Could you check a few things on this model? Use its own coordinates, in mm. Face numbers are marked on the shaded views. A direction names the side the tool comes from. Give positions to 0.01 mm unless a question says otherwise; leave off trailing zeros. Loops run counter-clockwise (first coordinate to the right, second up) from the corner with the lowest first, then second, coordinate; pieces in that order, holes last. Notation, with made-up numbers: M 55,27 L 109,27 A21 cw 109,35 Z; hole C 50.25,-16.75 d1. An arc over 180 degrees is marked long. Return JSON: item names as keys, results as strings. Group by question number.
1. For the marked faces 4 and 5, which set-ups out of +Z, -Z, +X, -X, +Y, -Y let a thin tool reach every point of the face, with its end or its side?
2. Please list where these lines run through material, in increasing order: line 1 (Z direction, x = 5.75, y = -4.75); line 2 (Z direction, x = -3, y = -7); line 3 (Z direction, x = 2.75, y = 11.5).
3. If we mould it in two halves opening along Z, with no side actions, what happens to the marked faces 1, 2 and 3? For each: +Z half, -Z half, draft (parallel to the pull), parting line (faces both ways), or undercut.
4. If we section it at A-A (z = 0.5): Write out the boundary of the cut face in (x, y), plus the area to 3 significant figures.
5. For pin 1 (1.4 mm diameter, centred on x = -11.5, y = 6, fed in from -Z); pin 2 (1.6 mm diameter, centred on x = -11.5, y = -6.5, fed in from -Z); pin 3 (0.8 mm diameter, centred on x = -7.5, z = -2, fed in from -Y); pin 4 (3 mm diameter, centred on x = -11, y = 6, fed in from +Z), each with a flat end and sliding along its axis, tell me the tip position at first contact or that it passes through.
```python
from build123d import *

# Parameters (mm, degrees)
EXTRUDE_1_DEPTH     = 9.5
SKETCH_6_R          = 7
EXTRUDE_2_DEPTH     = 13.5
SWEEP_1_PITCH       = 4
SWEEP_1_HEIGHT      = 10
SWEEP_1_RADIUS      = 7
REVOLVE_2_ANGLE     = 45
CHAMFER_1_SIZE      = 1
CUT_EXTRUDE_2_DEPTH = 0.4
SKETCH_13_R         = 2.5
CUT_EXTRUDE_3_DEPTH = 0.4
CUT_EXTRUDE_4_DEPTH = 0.4
SKETCH_14_W         = 5
SKETCH_14_H         = 5
CUT_EXTRUDE_5_DEPTH = 0.4


with BuildPart() as part:
    # 草图1 → 凸台-拉伸1 (new body)
    with BuildSketch(Plane.XY):
        Polygon((15, 0), (7.5, 12.990381057), (-7.5, 12.990381057), (-15, 0), (-7.5, -12.990381057), (7.5, -12.990381057), align=None)
    extrude(amount=EXTRUDE_1_DEPTH)

    # 草图6 → 凸台-拉伸2 (add)
    with BuildSketch(Plane(origin=(0, 0, 0), x_dir=(-1, 0, 0), z_dir=(0, 0, -1))):
        Circle(SKETCH_6_R)
    extrude(amount=EXTRUDE_2_DEPTH)

    # 扫描1: sweep along a helix
    with BuildLine() as sweep_1_path:
        Helix(SWEEP_1_PITCH, SWEEP_1_HEIGHT, SWEEP_1_RADIUS, center=(0, 0, -1.75), direction=(0, 0, -1))
    # 草图8 → 扫描1 (sweep)
    with BuildSketch(Plane(origin=(0, 0, 0), x_dir=(1, 0, 0), z_dir=(0, 1, 0))):
        Polygon((-7, 3.5), (-7, 0), (-8.5, 1.5), (-8.5, 2), align=None)
    sweep(path=sweep_1_path.line, is_frenet=True)

    # 草图9 → 旋转2 (revolve)
    with BuildSketch(Plane(origin=(0, 0, 0), x_dir=(1, 0, 0), z_dir=(0, 1, 0))):
        Polygon((7, 3.5), (7, 0), (8.5, 1.5), (8.5, 2), align=None)
    revolve(axis=Axis((0, 0, 0), (0, 0, 1)), revolution_arc=REVOLVE_2_ANGLE)

    # 倒角1
    chamfer_1_edges = [part.edges().sort_by_distance(p)[0] for p in [
        (-11.25, 6.495190528, 9.5),
        (-11.25, -6.495190528, 9.5),
        (0, -12.990381057, 9.5),
        (11.25, -6.495190528, 9.5),
        (11.25, 6.495190528, 9.5),
        (11.25, -6.495190528, 0),
        (0, -12.990381057, 0),
        (-11.25, -6.495190528, 0),
        (-11.25, 6.495190528, 0),
        (0, 12.990381057, 0),
        (11.25, 6.495190528, 0),
        (0, 12.990381057, 9.5),
    ]]
    chamfer(chamfer_1_edges, length=CHAMFER_1_SIZE)

    # 草图11 → 切除-拉伸2 (cut)
    with BuildSketch(Plane(origin=(-11.25, -6.495190528, 0), x_dir=(0, 0, 1), z_dir=(-0.8660254037844389, -0.4999999999999995, 0))):
        Polygon((2.25, 0), (7.25, 2.886751346), (7.25, -2.886751346), align=None)
    extrude(amount=-CUT_EXTRUDE_2_DEPTH, mode=Mode.SUBTRACT)

    # 草图13 → 切除-拉伸3 (cut)
    with BuildSketch(Plane(origin=(11.25, -6.495190528, 0), x_dir=(0, 0, -1), z_dir=(0.8660254037844387, -0.5000000000000001, 0))):
        with Locations(Location((-4.75, 0, 0), (0, 0, 90))):
            Circle(SKETCH_13_R)
    extrude(amount=-CUT_EXTRUDE_3_DEPTH, mode=Mode.SUBTRACT)

    # 草图12 → 切除-拉伸4 (cut)
    with BuildSketch(Plane.XZ.offset(12.990381057)):
        Polygon((-2.5, 6.825735931), (2.075735931, 2.25), (2.5, 2.674264069), (-2.075735931, 7.25), align=None)
        Polygon((2.075735931, 7.25), (-2.5, 2.674264069), (-2.075735931, 2.25), (2.5, 6.825735931), align=None)
    extrude(amount=-CUT_EXTRUDE_4_DEPTH, mode=Mode.SUBTRACT)

    # 草图14 → 切除-拉伸5 (cut)
    with BuildSketch(Plane(origin=(-11.25, 6.495190528, 0), x_dir=(0, 0, 1), z_dir=(-0.8660254037844384, 0.5000000000000006, 0))):
        with Locations((4.75, 0)):
            Rectangle(SKETCH_14_W, SKETCH_14_H)
    extrude(amount=-CUT_EXTRUDE_5_DEPTH, mode=Mode.SUBTRACT)


solid = part.part
```
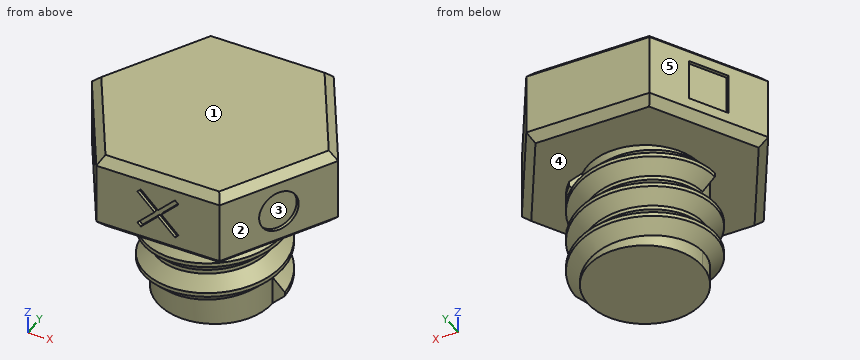
Answer:
{
 "1": {"face 4": "none", "face 5": "+Z, -Z, -X, +Y"},
 "2": {"line 1": "z = -9.48 to -6.9, -5.48 to -2.9, 0 to 9.5", "line 2": "z = -10.14 to -7.87, -6.14 to -3.87, 0 to 9.5", "line 3": "z = 0 to 9.5"},
 "3": {"face 1": "+Z half", "face 2": "draft", "face 3": "undercut"},
 "4": {"outline": "M -14.42,0 L -7.21,-12.49 L 7.21,-12.49 L 14.42,0 L 7.21,12.49 L -7.21,12.49 Z", "area": "540 mm²"},
 "5": {"pin 1": "stops at z = 0.27", "pin 2": "stops at z = 0.42", "pin 3": "stops at y = 0", "pin 4": "stops at z = 9.5"}
}
